The listing builds one solid part. Answer for the finished solid, in the listing's coordinates (mm). A direction names the side the tool comes from. Give positions to 0.01 mm unless a question says otherwise; leave off trailing zeros. Write each loop counter-clockwise with the first axis right and the second up, starting at its lowest first coordinate (ties: lowest second). Pieces come first, ordered by that corner, then holes. Notation, with made-up numbers: (7.25, 47) -> (47.25, 47) arc R24 ccw to (47.25, 80) -> close; hole circle Ø4 at (-27.75, 2). An arc over 180 degrees is marked (long way). Use CSV: the item, a comma, the result in double quotes. Start each with the question number.
from build123d import *


with BuildPart() as f2:
    # F2: sweep along a path in F1
    with BuildLine(Plane.XZ) as f2_path:
        ThreePointArc((0, 0), (-17.046052, 32.711514), (-53.622998, 37.479948))
        Line((-53.622998, 37.479948), (-156.060986, 0))
    # F0 (on Top) → F2 (sweep)
    with BuildSketch(Plane.XY):
        Polygon((-12.949203, 16.38248), (-20.740632, 2.427694), (-16.38248, -12.949203), (-2.427694, -20.740632), (12.949203, -16.38248), (20.740632, -2.427694), (16.38248, 12.949203), (2.427694, 20.740632), align=None)
    sweep(path=f2_path.line)


solid = f2.part
Q1. Section B-B on y = -7 is taken. Give the vertices of the cut face in (x, z).
Q2. Flat-ended cylindrical pins translate along their axes: pin 1 Ø2 at (x, y) = (-87.5, 13.5) entering from -Z; pin 2 Ø8 at (y, z) = (8.5, 50) entering from +X; pin 3 Ø2 at (x, y) = (-78.5, 13) entering from +Z; pin 4 Ø2 at (x, z) = (-125.5, 36) entering from +Y (3 decimals). Find the tip coordinate at first contact, or state that the pin passes through.
Q3. Section D-D on y = 5.5 is taken. Give the vertices of the cut face in (x, z).
Q4. Straight lines are drawn through the part: L1, parallel to Z at x = -52, y = 15; L2, parallel to Y at x = 12.5, z = 1.5; L3, parallel to Z at x = -14, y = -10. For each, find the intervals that lie inside material, in ascending order.
Q5. The mould has two halves that part along X. Classify faces 1 (the face through (-111.328, -9.503, 34.246)), 2 (the face through (-99.79, 9.5, 2.71)), 3 (the face through (-7.752, -12.408, 44.715)): +X half, -X half, draft (parallel to the pull), parting line (faces both ways), or undercut.
Q6. For faces 4 (the face through (-111.947, 5.153, 35.938)), 5 (the face through (0, 0, 0)), 6 (the face through (-99.171, -5.153, 1.018)), 7 (the face through (-107.3, -18.6, 23.3)), 8 (the face through (-103.788, 18.592, 13.638)), determine the directions among +Z, -Z, +X, -X, +Y, -Y from which every point of the face is accessible in a straight line to the end or side of a thin tool.
Q7. Section C-C on z = -9 is taken. Give the vertices of the cut face in (x, y).
Q8. Section A-A on x = -84.5 is taken. Give the vertices of the cut face in (y, z), then the cut area to 3 significant figures.
Output:
1,outline,"(-162.31, 17.08) -> (-149.85, -16.97) -> (-47.41, 20.51) arc R21.84 cw to (-18.07, 0) -> (18.19, 0) arc R58.1 ccw to (-59.87, 54.56) -> close"
2,pin 1,"z = 8.88"
2,pin 2,"x = -5"
2,pin 3,"z = 46.28"
2,pin 4,"through"
3,outline,"(-162.42, 17.37) -> (-149.52, -17.87) -> (-47.09, 19.61) arc R20.88 cw to (-19.03, 0) -> (18.49, 0) arc R58.4 ccw to (-59.98, 54.85) -> close"
4,L1,"23.46 to 51.21"
4,L2,"-16.5 to 15.1"
4,L3,"0 to 50.12"
5,face 1,"-X half"
5,face 2,"undercut"
5,face 3,"parting line"
6,face 4,"+Z, -X, +Y"
6,face 5,"-Z, +X, +Y, -Y"
6,face 6,"-Z, -Y"
6,face 7,"+Z, -X, -Y"
6,face 8,"-Z, +Y"
7,outline,"(-152.77, -16.75) -> (-132.98, -12.95) -> (-120.3, 2.43) -> (-142.97, 16.38) -> (-152.77, 17.34) -> close"
8,outline,"(-20.74, 23.6) -> (-12.95, 8.74) -> (2.43, 4.1) -> (16.38, 12.39) -> (20.74, 28.77) -> (12.95, 43.63) -> (-2.43, 48.27) -> (-16.38, 39.97) -> close"
8,area,"1,310 mm²"
